Job drawing, mm, ordinate dimensions from the low corner. One solid piece. Give positions to 0.01 mm unless a question says otherwise; leave off trailing zeros. Order: outer loops, then holes, each group sorted by start corner. A loop starts at its lowest first (then second) coordinate and runs counter-clockwise, first axis right, second up.
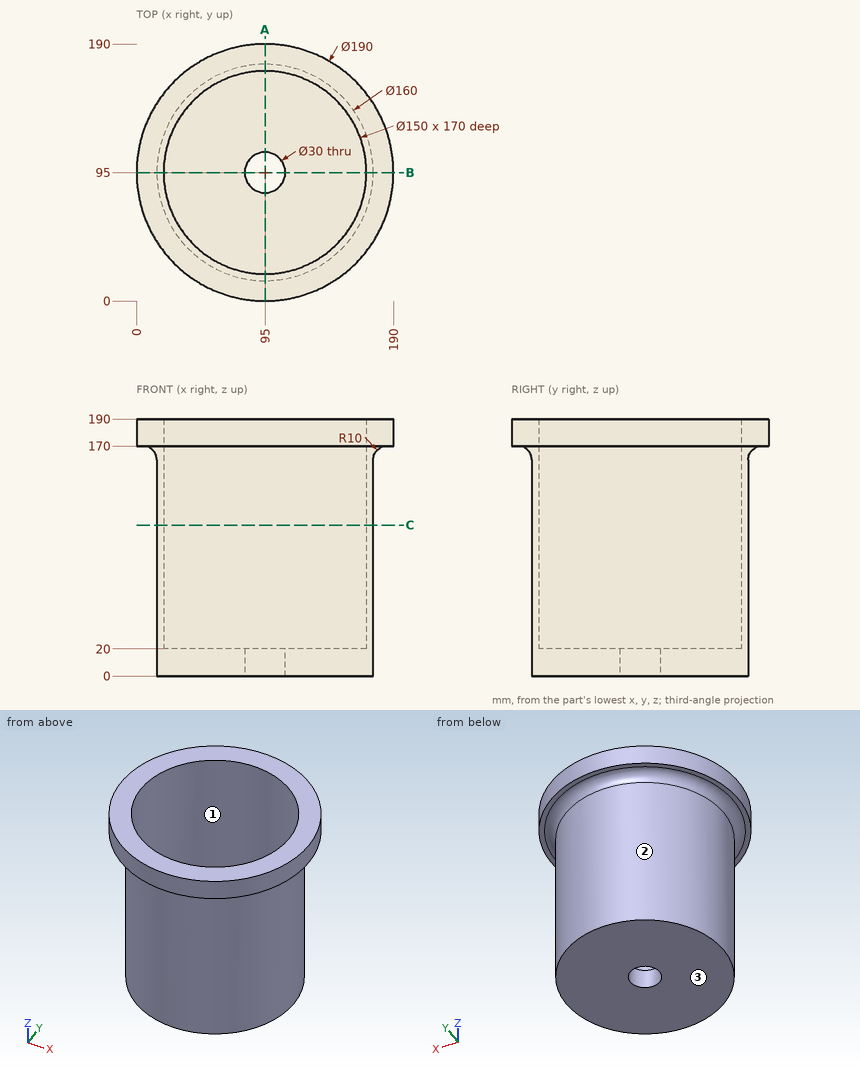
Item 1: Drop flat-ended pins along their axis: P1, Ø1.5, axis at x = 124.5, z = 66.5, coming from the +Y side; P2, Ø1, axis at x = 100, z = 133, coming from the -Y side; P3, Ø12, axis at x = 95.5, z = 46.5, coming from the -Y side. Give the stop position or say it passes through.
Item 2: Pull direction Y, two halves, no side cores. Call the marked faces 1, 2 and 3: released by +Y, released by -Y, zero draft, split by the parting line, or undercut.
Item 3: Drill centre lines: probe 1 along Z at (x, y) = (90, 146.5); probe 2 along X at (y, z) = (32, 38); probe 3 along Y at (x, z) = (28.5, 152.5). Where is each one in solid material? Low to high.
Item 4: Band-saw the part on A-A on x = 95. List the corners of the cut face in (y, z), plus the area to 3 significant figures.
Item 5: Band-saw the part on C-C on z = 111.5. List the corners of the cut face in (x, y).
Working result:
1. P1: stops at y = 169.66
1. P2: stops at y = 15.13
1. P3: stops at y = 15
2. face 1: undercut
2. face 2: split by the parting line
2. face 3: zero draft
3. probe 1: z = 0 to 20
3. probe 2: x = 45.69 to 54.31, 135.69 to 144.31
3. probe 3: y = 50.53 to 60.32, 129.68 to 139.47
4. outline: (0, 170) - (5, 170) arc R10 cw to (15, 160) - (15, 0) - (80, 0) - (80, 20) - (20, 20) - (20, 190) - (0, 190) - close; (110, 0) - (175, 0) - (175, 160) arc R10 cw to (185, 170) - (190, 170) - (190, 190) - (170, 190) - (170, 20) - (110, 20) - close
4. area: 4,940 mm2
5. outline: circle Ø160 at (95, 95); hole circle Ø150 at (95, 95)
